Can you work these out from the model? Positions are in its coordinate system, mm. Round coordinates to 2 decimals unless told otherwise and drop trailing zeros. Loops run counter-clockwise (first coordinate to the right, second up) from the corner with the lowest first, then second, coordinate; pieces in that order, holes last.
from build123d import *

# Parameters (mm, degrees)
EXTRUDE1_DEPTH             = 390
EXTRUDE2_REACH             = 392.08
SKETCH2_R                  = 1.75
SKETCH_R                   = 3
SKETCH_R_2                 = 1.75
EXTRUDE4_DEPTH             = 3.5
CHAMFER1_SIZE              = 0.2
LPATTERN1_COUNT            = 19
LPATTERN1_PITCH            = 20
CHAMFER1_OF_LPATTERN1_SIZE = 0.2


with BuildPart() as part:
    # Sketch1 → Extrude1 (new body)
    with BuildSketch(Plane.XY):
        with BuildLine():
            Line((-4.3, -3.25), (4.3, -3.25))
            Line((4.3, -3.25), (4.5, -3.05))
            Line((4.5, -3.05), (4.5, 0.455012563))
            ThreePointArc((4.5, 0.455012563), (3.924845827, 0.712323349), (3.617735397, 1.2625))
            Line((3.617735397, 1.2625), (3.15008224, 1.2625))
            Line((3.15008224, 1.2625), (3.15008224, 1.7625))
            Line((3.15008224, 1.7625), (3.65008224, 1.7625))
            ThreePointArc((3.65008224, 1.7625), (3.973877727, 2.229724887), (4.5, 2.444987437))
            Line((4.5, 2.444987437), (4.5, 3.05))
            Line((4.5, 3.05), (4.3, 3.25))
            Line((4.3, 3.25), (-4.3, 3.25))
            Line((-4.3, 3.25), (-4.5, 3.05))
            Line((-4.5, 3.05), (-4.5, 2.444987437))
            ThreePointArc((-4.5, 2.444987437), (-3.973877727, 2.229724887), (-3.65008224, 1.7625))
            Line((-3.65008224, 1.7625), (-3.15008224, 1.7625))
            Line((-3.15008224, 1.7625), (-3.15008224, 1.2625))
            Line((-3.15008224, 1.2625), (-3.617735397, 1.2625))
            ThreePointArc((-3.617735397, 1.2625), (-3.924845827, 0.712323349), (-4.5, 0.455012563))
            Line((-4.5, 0.455012563), (-4.5, -3.05))
            Line((-4.5, -3.05), (-4.3, -3.25))
        make_face()
    extrude(amount=EXTRUDE1_DEPTH)

    # Sketch2 → Extrude2 (cut, up to next)
    with BuildSketch(Plane(origin=(0, 3.25, 0), x_dir=(1, 0, 0), z_dir=(0, 1, 0)), mode=Mode.PRIVATE) as extrude2_sk1:
        with Locations(Location((0, -15, 0), (0, 0, 270))):
            Circle(SKETCH2_R)
    extrude2_tool1 = extrude(extrude2_sk1.sketch, amount=-EXTRUDE2_REACH, mode=Mode.PRIVATE) & part.part
    extrude2 = extrude2_tool1.solids().sort_by_distance((0, 3.25, 15))[0]
    add(extrude2, mode=Mode.SUBTRACT)

    # Sketch → Extrude4 (cut)
    with BuildSketch(Plane(origin=(0, 3.25, 0), x_dir=(1, 0, 0), z_dir=(0, 1, 0))):
        with Locations(Location((0, -15, 0), (0, 0, 270))):
            Circle(SKETCH_R)
        with Locations(Location((0, -15, 0), (0, 0, 270))):
            Circle(SKETCH_R_2, mode=Mode.SUBTRACT)
    extrude4 = extrude(amount=-EXTRUDE4_DEPTH, mode=Mode.SUBTRACT)

    # Chamfer1
    chamfer1_edges = [part.edges().sort_by_distance(p)[0] for p in [
        (0, -3.25, 13.25),
        (0, 3.25, 12),
    ]]
    chamfer(chamfer1_edges, length=CHAMFER1_SIZE)

    # LPattern1: Extrude2, Extrude4 ×19
    with Locations(*[(0, 0, i * LPATTERN1_PITCH) for i in range(1, LPATTERN1_COUNT)]):
        add(extrude2, mode=Mode.SUBTRACT)
        add(extrude4, mode=Mode.SUBTRACT)

    # Chamfer1 of LPattern1
    chamfer1_of_lpattern1_edges = [part.edges().sort_by_distance(p)[0] for p in [
        (0, -3.25, 33.25),
        (0, 3.25, 32),
        (0, -3.25, 53.25),
        (0, 3.25, 52),
        (0, -3.25, 73.25),
        (0, 3.25, 72),
        (0, -3.25, 93.25),
        (0, 3.25, 92),
        (0, -3.25, 113.25),
        (0, 3.25, 112),
        (0, -3.25, 133.25),
        (0, 3.25, 132),
        (0, -3.25, 153.25),
        (0, 3.25, 152),
        (0, -3.25, 173.25),
        (0, 3.25, 172),
        (0, -3.25, 193.25),
        (0, 3.25, 192),
        (0, -3.25, 213.25),
        (0, 3.25, 212),
        (0, -3.25, 233.25),
        (0, 3.25, 232),
        (0, -3.25, 253.25),
        (0, 3.25, 252),
        (0, -3.25, 273.25),
        (0, 3.25, 272),
        (0, -3.25, 293.25),
        (0, 3.25, 292),
        (0, -3.25, 313.25),
        (0, 3.25, 312),
        (0, -3.25, 333.25),
        (0, 3.25, 332),
        (0, -3.25, 353.25),
        (0, 3.25, 352),
        (0, -3.25, 373.25),
        (0, 3.25, 372),
    ]]
    chamfer(chamfer1_of_lpattern1_edges, length=CHAMFER1_OF_LPATTERN1_SIZE)


solid = part.part
(1) If we section it at B-B, the plane z = 204.5: List the corners of the cut face in (x, y) for me, then the cut area to 3 significant figures.
Worked answers:
outline: (-4.5, -3.05) - (-4.3, -3.25) - (4.3, -3.25) - (4.5, -3.05) - (4.5, 0.46) arc R1 cw to (3.62, 1.26) - (3.15, 1.26) - (3.15, 1.76) - (3.65, 1.76) arc R1 cw to (4.5, 2.44) - (4.5, 3.05) - (4.3, 3.25) - (-4.3, 3.25) - (-4.5, 3.05) - (-4.5, 2.44) arc R1 cw to (-3.65, 1.76) - (-3.15, 1.76) - (-3.15, 1.26) - (-3.62, 1.26) arc R1 cw to (-4.5, 0.46) - close
area: 55.2 mm2
(2) If I drill on line 1 (X direction, y = -2.2, z = 215); line 2 (Y direction, x = 3.5, z = 192.5); line 3 (Y direction, x = 1.5, z = 36), over which ranges is the centre line in solid material (lowest first)?
Worked answers:
line 1: x = -4.5 to -1.75, 1.75 to 4.5
line 2: y = -3.25 to 1.26, 1.76 to 3.25
line 3: y = -3.1 to -0.25
(3) If we mould it in two halves opening along Z, with no side actions, what happens to faces 1 (the flat face through (0, -3.25, 192)), 2 (the flat face through (0, -0.25, 237))? For each: released by +Z, released by -Z, zero draft, split by the parting line, or undercut.
Worked answers:
face 1: zero draft
face 2: undercut
(4) If we section it at A-A, the plane y = -1.5: State how many separate pieces and enclosed holes the cut face has, then the cut area to 3 significant figures.
Worked answers:
separate pieces: 1
enclosed holes: 19
area: 3,330 mm2
(5) Will this pin go through, and if not, where does the flat tip stop? P1, Ø3, axis at x = 1, z = 174, coming from the +Y side.
Worked answers:
P1: stops at y = -0.25
